CAD build for the part. Positions are in the model's coordinates, mm. A direction names the side the tool comes from. Coordinates: 2 decimals unless noted, no trailing zeros. Order: outer loops, then holes, each group sorted by start corner. A loop starts at its lowest first (then second) coordinate and runs counter-clockwise, first axis right, second up. Notation, with made-up numbers: (-19.5, 50.5) - (39.5, 50.5) arc R24 ccw to (39.5, 71.5) - close; hole circle Ø4 at (21, 89.5). An arc over 180 degrees is marked (long way). Write each question's results on one line, items separated by ' | '. Start each with the question number.
Q1. Band-saw the part on B-B, the plane y = 35. Write the cut outline in (x, z).
Q2. Pin check, flat tips, straight feed: P1, Ø5, axis at x = 77.5, y = -35, coming from the -Z side; P2, Ø7, axis at x = -77.5, y = 35, coming from the -Z side. Stop position of each tip, or through.
Q3. Which spindle directions (+Z, -Z, +X, -X, +Y, -Y) get a long thin tool onto all of the face, cutting with end or side? Do faces 1 (the flat face through (-1, 35, 3)), 2 (the flat face through (-1, -54, 0)). Say none if no direction does.
Q4. Band-saw the part on A-A, the plane x = -77.5. Write the cut outline in (y, z).
Q5. Band-saw the part on C-C, the plane x = 62.5. Write the cut outline in (y, z).
Q6. Pull direction X, two halves, no side cores. Call faces 3 (the flat face through (-85, -1, 4)), 4 (the flat face through (-1, 0, 0)), 5 (the cylindrical face through (45.5, 49.67, 5.46)): released by +X, released by -X, zero draft, split by the parting line, or undercut.
Q7. Band-saw the part on D-D, the plane x = -33.5. Write the cut outline in (y, z), then the cut area to 3 significant figures.
Q8. Wall check: probe 1 along X at (y, z) = (35, 4.15); probe 2 along Y at (x, z) = (-62.5, 3.8); probe 3 along Y at (x, z) = (11, 1.5). Give the ranges that are in metal, low to high.
```python
from build123d import *

# Parameters (mm, degrees)
F0_W          = 170
F0_H          = 140
F0_R          = 4
F1_DEPTH      = 8
F2_SIZE       = 3
F3_W          = 180
F3_H          = 10
F4_DEPTH      = 25
F4_DEPTH_BACK = 3
F5_R          = 3
F6_DEPTH      = 25
F7_SIZE       = 2.5
F8_SIZE       = 0.6


with BuildPart() as f1:
    # F0 (on Top) → F1 (new body)
    with BuildSketch(Plane.XY):
        Rectangle(F0_W, F0_H)
        with Locations((-49.4974746831, -49.4974746831)):
            Circle(F0_R, mode=Mode.SUBTRACT)
        with Locations((49.4974746831, -49.4974746831)):
            Circle(F0_R, mode=Mode.SUBTRACT)
        with Locations((-49.4974746831, 49.4974746831)):
            Circle(F0_R, mode=Mode.SUBTRACT)
        with Locations((49.4974746831, 49.4974746831)):
            Circle(F0_R, mode=Mode.SUBTRACT)
    extrude(amount=F1_DEPTH)

    # F2
    f2_edges = [f1.edges().sort_by_distance(p)[0] for p in [
        (-53.497475, -49.497475, 0),
        (-53.497475, 49.497475, 0),
        (45.497475, 49.497475, 0),
        (45.497475, -49.497475, 0),
    ]]
    chamfer(f2_edges, length=F2_SIZE)

    # F3 (on Top) → F4 (cut, two sides)
    with BuildSketch(Plane.XY) as f4_sk:
        with Locations((0, -35)):
            Rectangle(F3_W, F3_H)
        with Locations((0, 35)):
            Rectangle(F3_W, F3_H)
    extrude(amount=-F4_DEPTH, mode=Mode.SUBTRACT)
    extrude(f4_sk.sketch, amount=F4_DEPTH_BACK, mode=Mode.SUBTRACT)

    # F5 (on Top) → F6 (cut)
    with BuildSketch(Plane.XY):
        with Locations((-62.5, -35)):
            Circle(F5_R)
        with Locations((-77.5, -35)):
            Circle(F5_R)
        with Locations((-62.5, 35)):
            Circle(F5_R)
        with Locations((-77.5, 35)):
            Circle(F5_R)
        with Locations((62.5, 35)):
            Circle(F5_R)
        with Locations((77.5, 35)):
            Circle(F5_R)
        with Locations((62.5, -35)):
            Circle(F5_R)
        with Locations((77.5, -35)):
            Circle(F5_R)
    extrude(amount=F6_DEPTH, mode=Mode.SUBTRACT)

    # F7
    f7_edges = [f1.edges().sort_by_distance(p)[0] for p in [
        (-65.5, 35, 8),
        (-65.5, -35, 8),
        (59.5, -35, 8),
        (59.5, 35, 8),
    ]]
    chamfer(f7_edges, length=F7_SIZE)

    # F8
    f8_edges = [f1.edges().sort_by_distance(p)[0] for p in [
        (-85, 0, 8),
        (0, 70, 8),
        (0, -70, 8),
        (85, 0, 8),
        (85, -70, 4),
        (-85, -70, 4),
        (85, 55, 0),
        (-85, 55, 0),
        (0, 70, 0),
        (-85, 0, 0),
        (-85, -55, 0),
        (85, 0, 0),
        (85, -55, 0),
        (0, -70, 0),
        (85, 70, 4),
        (-85, 70, 4),
    ]]
    chamfer(f8_edges, length=F8_SIZE)


solid = f1.part
```
Results below:
1) outline: (-85, 3) - (-80.5, 3) - (-80.5, 8) - (-84.4, 8) - (-85, 7.4) - close; (-74.5, 3) - (-65.5, 3) - (-65.5, 5.5) - (-68, 8) - (-74.5, 8) - close; (-59.5, 3) - (59.5, 3) - (59.5, 5.5) - (57, 8) - (-57, 8) - (-59.5, 5.5) - close; (65.5, 3) - (74.5, 3) - (74.5, 8) - (68, 8) - (65.5, 5.5) - close; (80.5, 3) - (85, 3) - (85, 7.4) - (84.4, 8) - (80.5, 8) - close
2) P1: passes through | P2: stops at z = 3
3) face 1: -Z, +X, -X | face 2: -Z, +X, -X, +Y, -Y
4) outline: (-70, 0.6) - (-69.4, 0) - (-40, 0) - (-40, 3) - (-38, 3) - (-38, 8) - (-69.4, 8) - (-70, 7.4) - close; (-32, 3) - (-30, 3) - (-30, 0) - (30, 0) - (30, 3) - (32, 3) - (32, 8) - (-32, 8) - close; (38, 3) - (40, 3) - (40, 0) - (69.4, 0) - (70, 0.6) - (70, 7.4) - (69.4, 8) - (38, 8) - close
5) outline: (-70, 0.6) - (-69.4, 0) - (-40, 0) - (-40, 3) - (-38, 3) - (-38, 5.5) - (-40.5, 8) - (-69.4, 8) - (-70, 7.4) - close; (-32, 3) - (-30, 3) - (-30, 0) - (30, 0) - (30, 3) - (32, 3) - (32, 5.5) - (29.5, 8) - (-29.5, 8) - (-32, 5.5) - close; (38, 3) - (40, 3) - (40, 0) - (69.4, 0) - (70, 0.6) - (70, 7.4) - (69.4, 8) - (40.5, 8) - (38, 5.5) - close
6) face 3: released by -X | face 4: zero draft | face 5: undercut
7) outline: (-70, 0.6) - (-69.4, 0) - (-40, 0) - (-40, 3) - (-30, 3) - (-30, 0) - (30, 0) - (30, 3) - (40, 3) - (40, 0) - (69.4, 0) - (70, 0.6) - (70, 7.4) - (69.4, 8) - (-69.4, 8) - (-70, 7.4) - close | area: 1,060 mm²
8) probe 1: x = -85 to -80.5, -74.5 to -65.5, -59.5 to 59.5, 65.5 to 74.5, 80.5 to 85 | probe 2: y = -70 to -38, -32 to 32, 38 to 70 | probe 3: y = -70 to -40, -30 to 30, 40 to 70
